CAD build for the part. Positions are in the model's coordinates, mm. A direction names the side the tool comes from. Give positions to 0.01 mm unless a question says otherwise; leave off trailing zeros. Loops run counter-clockwise (first coordinate to the right, second up) from the corner with the lowest first, then second, coordinate; pieces in that order, holes last. Notation, with made-up numbers: (7.25, 7) - (27.25, 7) arc R15 ccw to (27.25, 15) - close; hole circle Ø3 at (84.25, 59). An arc over 180 degrees is marked (long way). Return JSON: item names as keys, results as strings.
from build123d import *

# Parameters (mm, degrees)
F0_R     = 6.35
F1_DEPTH = 25.4
F3_DEPTH = 6.35
F5_DEPTH = 6.35
F7_DEPTH = 25.4
F9_DEPTH = 25.4


# Not quite as in the source:
# - a pattern or mirror of a feature is missing from the dataset's text; its kind, count and spacing are read off the source's solid
# - a feature names something its author has since deleted; it is built from what else it names


with BuildPart() as f1:
    # F0 (on Front) → F1 (new body)
    with BuildSketch(Plane.XZ):
        Polygon((0, 25.4), (0, 0), (12.7, 0), (12.7, 19.05), (12.7, 25.4), align=None)
        with BuildLine():
            Line((12.7, 19.05), (12.7, 0))
            Line((12.7, 0), (28.575, 0))
            ThreePointArc((28.575, 0), (19.05, 9.525), (28.575, 19.05))
            Line((28.575, 19.05), (12.7, 19.05))
        make_face()
        with BuildLine():
            ThreePointArc((28.575, 19.05), (19.05, 9.525), (28.575, 0))
            ThreePointArc((28.575, 0), (35.3101920908, 2.7898079092), (38.1, 9.525))
            ThreePointArc((38.1, 9.525), (35.3101920908, 16.2601920908), (28.575, 19.05))
        make_face()
        with Locations((28.575, 9.525)):
            Circle(F0_R, mode=Mode.SUBTRACT)
    extrude(amount=F1_DEPTH)

    # F2 (on face) → F3 (cut)
    with BuildSketch(Plane.XZ):
        with BuildLine():
            Line((28.575, 19.05), (12.7, 19.05))
            Line((12.7, 19.05), (12.7, 0))
            Line((12.7, 0), (28.575, 0))
            ThreePointArc((28.575, 0), (19.05, 9.525), (28.575, 19.05))
        make_face()
    extrude(amount=-F3_DEPTH, mode=Mode.SUBTRACT)

    # F4 (on Front) → F5 (cut)
    with BuildSketch(Plane.XZ):
        with BuildLine():
            Line((28.575, 19.05), (12.7, 19.05))
            Line((12.7, 19.05), (12.7, 0))
            Line((12.7, 0), (28.575, 0))
            ThreePointArc((28.575, 0), (19.05, 9.525), (28.575, 19.05))
        make_face()
    f5 = extrude(amount=F5_DEPTH, mode=Mode.SUBTRACT)

    # F5_copies: F5 across plane
    add(f5.mirror(Plane(origin=(0, -12.7, 0), x_dir=(0, 0, -1), z_dir=(0, -1, 0))), mode=Mode.SUBTRACT)

    # F6 (on Right) → F7 (cut)
    with BuildSketch(Plane.YZ):
        Polygon((-25.4, 19.05), (-19.05, 25.4), (-25.4, 25.4), align=None)
    extrude(amount=F7_DEPTH, mode=Mode.SUBTRACT)

    # F8 (on Right) → F9 (cut)
    with BuildSketch(Plane.YZ):
        Polygon((0, 19.05), (0, 25.4), (-6.35, 25.4), align=None)
    extrude(amount=F9_DEPTH, mode=Mode.SUBTRACT)


solid = f1.part
1. Which spindle directions (+Z, -Z, +X, -X, +Y, -Y) get a long thin tool onto all of the face, cutting with end or side? Do faces 5 (the face through (22.23, -12.52, 9.8)), 6 (the face through (38.02, -12.52, 10.76)). Say none if no direction does.
Values follow:
{"face 5": "+Y, -Y", "face 6": "none"}
2. Cut at C-C, the plane x = 7. Write the cut outline in (y, z).
Values follow:
{"outline": "(-25.4, 0) - (0, 0) - (0, 19.05) - (-6.35, 25.4) - (-19.05, 25.4) - (-25.4, 19.05) - close"}
3. Drill centre lines: probe 1 along X at (y, z) = (-17.5, 9.5); probe 2 along X at (y, z) = (-2.5, 14.5); probe 3 along X at (y, z) = (-19.5, 15). Where is each one in solid material? Low to high.
Values follow:
{"probe 1": "x = 0 to 22.23, 34.92 to 38.1", "probe 2": "x = 0 to 12.7, 20.45 to 24.63, 32.52 to 36.7", "probe 3": "x = 0 to 12.7, 20.78 to 25.36, 31.79 to 36.37"}
4. Cut at D-D, the plane x = 32.5. Write the cut outline in (y, z), plus the area to 3 significant figures.
Values follow:
{"outline": "(-25.4, 0.85) - (0, 0.85) - (0, 4.53) - (-25.4, 4.53) - close; (-25.4, 14.52) - (0, 14.52) - (0, 18.2) - (-25.4, 18.2) - close", "area": "187 mm²"}
5. Pull direction X, two halves, no side cores. Call faces 1 (the face through (0, -13, 13)), 2 (the face through (12.7, -13, 21)), 3 (the face through (21, -13, 19.05)), 4 (the face through (17, -19.05, 10)): +X half, -X half, draft (parallel to the pull), parting line (faces both ways), or undercut.
Values follow:
{"face 1": "-X half", "face 2": "undercut", "face 3": "draft", "face 4": "undercut"}
6. Cut at B-B, the plane z = 13.5. Write the cut outline in (x, y), plus the area to 3 significant figures.
Values follow:
{"outline": "(0, -25.4) - (12.7, -25.4) - (12.7, -19.05) - (19.92, -19.05) - (19.92, -25.4) - (23.62, -25.4) - (23.62, 0) - (19.92, 0) - (19.92, -6.35) - (12.7, -6.35) - (12.7, 0) - (0, 0) - close; (33.53, -25.4) - (37.23, -25.4) - (37.23, 0) - (33.53, 0) - close", "area": "602 mm²"}
7. Drop flat-ended pins along their axis: P1, Ø1, axis at y = -21, z = 21, coming from the +X side; P2, Ø4, axis at y = -19.5, z = 3.5, coming from the +X side; P3, Ø4, axis at x = 19, y = -12, coming from the +Z side. Give the stop position or say it passes through.
Values follow:
{"P1": "stops at x = 12.7", "P2": "stops at x = 37.21", "P3": "stops at z = 19.05"}
8. Cut at A-A, the plane y = -4.75. Write the cut outline in (x, z) (3 decimals), plus the area to 3 significant figures.
Values follow:
{"outline": "(0, 0) - (12.7, 0) - (12.7, 23.8) - (0, 23.8) - close; circle Ø19.05 at (28.575, 9.525); hole circle Ø12.7 at (28.575, 9.525)", "area": "461 mm²"}
